```python
from build123d import *

# Parameters (mm, degrees)
SKETCH1_R           = 4.05
BOSS_EXTRUDE1_DEPTH = 16.8
SKETCH2_R           = 1
BOSS_EXTRUDE2_DEPTH = 0.3
SKETCH3_R           = 0.5
BOSS_EXTRUDE3_DEPTH = 4.7
SKETCH4_R           = 0.35
BOSS_EXTRUDE4_DEPTH = 5
FILLET1_R           = 0.5


with BuildPart() as part:
    # Sketch1 → Boss-Extrude1 (new body)
    with BuildSketch(Plane(origin=(0, 0, 0), x_dir=(0, 0, -1), z_dir=(1, 0, 0))):
        Circle(SKETCH1_R)
    extrude(amount=BOSS_EXTRUDE1_DEPTH)

    # Sketch2 → Boss-Extrude2 (add)
    with BuildSketch(Plane(origin=(16.8, 0, 0), x_dir=(0, 0, -1), z_dir=(1, 0, 0))):
        Circle(SKETCH2_R)
    extrude(amount=BOSS_EXTRUDE2_DEPTH)

    # Sketch3 → Boss-Extrude3 (add)
    with BuildSketch(Plane(origin=(17.1, 0, 0), x_dir=(0, 0, -1), z_dir=(1, 0, 0))):
        Circle(SKETCH3_R)
    extrude(amount=BOSS_EXTRUDE3_DEPTH)

    # Sketch4 → Boss-Extrude4 (add)
    with BuildSketch(Plane.ZY):
        with Locations(Location((2.4, 0, 0), (0, 0, 180))):
            Circle(SKETCH4_R)
        with Locations(Location((-2.4, 0, 0), (0, 0, 180))):
            Circle(SKETCH4_R)
    extrude(amount=BOSS_EXTRUDE4_DEPTH)

    # Fillet1
    fillet1_edges = [part.edges().sort_by_distance(p)[0] for p in [
        (16.8, 0, 4.05),
    ]]
    fillet(fillet1_edges, radius=FILLET1_R)


solid = part.part
```
Geometry check sheet. Reference: the model listing, model coordinates, mm. A direction names the side the tool comes from. Round coordinates to 2 decimals unless told otherwise and drop trailing zeros. Order: outer loops, then holes, each group sorted by start corner. A loop starts at its lowest first (then second) coordinate and runs counter-clockwise, first axis right, second up. Notation, with made-up numbers: (-8, 2) - (19, 2) arc R14 ccw to (19, 26) - close; hole circle Ø3 at (-31.75, 71). An arc over 180 degrees is marked (long way). Use a Markdown table: item, result. Add a question column.
1) Section check B-B (y = 0). Record the cut outline in (x, z).
2) Section check C-C (x = 7.75). Record the cut outline in (y, z).
3) Gauge pin test, flat ends, axial feed: P1, Ø2, axis at y = 0.5, z = 0.5, coming from the -X side; P2, Ø1.5, axis at x = 8.5, z = 2.5, coming from the -Y side; P3, Ø4, axis at x = 14.5, y = 1.5, coming from the +Z side; P4, Ø4, axis at y = 0.5, z = -3, coming from the +X side. Record the tip position at first contact, or that the pin passes through.
4) Thickness scan on line 1 along X through (y, z) = (0.5, -2.5); line 2 along Z through (x, y) = (8, -2.25); line 3 along Y through (x, z) = (4.5, 0.25). Record the ranges inside material, lowest first.
5) Set-up check for faces 1 (the cylindrical face through (8.036, -3.954, 0.878)), 2 (the flat face through (16.8, -1, -1)): record each of +Z, -Z, +X, -X, +Y, -Y from which the full face is reachable in a straight line by a thin tool's end or side.
6) Section check A-A (z = 0). Record the cut outline in (x, y), then the cut area to 3 significant figures.
Established:
| question | item | result |
|---|---|---|
| 1 | outline | (-5, -2.75) - (0, -2.75) - (0, -4.05) - (16.3, -4.05) arc R0.5 ccw to (16.8, -3.55) - (16.8, -1) - (17.1, -1) - (17.1, -0.5) - (21.8, -0.5) - (21.8, 0.5) - (17.1, 0.5) - (17.1, 1) - (16.8, 1) - (16.8, 3.55) arc R0.5 ccw to (16.3, 4.05) - (0, 4.05) - (0, 2.75) - (-5, 2.75) - (-5, 2.05) - (0, 2.05) - (0, -2.05) - (-5, -2.05) - close |
| 2 | outline | circle Ø8.1 at (0, 0) |
| 3 | P1 | x = 0 |
| 3 | P2 | y = -3.65 |
| 3 | P3 | z = 4.05 |
| 3 | P4 | x = 16.8 |
| 4 | line 1 | 0 to 16.8 |
| 4 | line 2 | -3.37 to 3.37 |
| 4 | line 3 | -4.04 to 4.04 |
| 5 | face 1 | +X, -X |
| 5 | face 2 | +X |
| 6 | outline | (0, -4.05) - (16.3, -4.05) arc R0.5 ccw to (16.8, -3.55) - (16.8, -1) - (17.1, -1) - (17.1, -0.5) - (21.8, -0.5) - (21.8, 0.5) - (17.1, 0.5) - (17.1, 1) - (16.8, 1) - (16.8, 3.55) arc R0.5 ccw to (16.3, 4.05) - (0, 4.05) - close |
| 6 | area | 141 mm2 |
